Verification items for the finished model (mm, model axes). Face numbers are marked on the shaded views. A direction names the side the tool comes from. Coordinates: 2 decimals unless noted, no trailing zeros. Loops run counter-clockwise (first coordinate to the right, second up) from the corner with the lowest first, then second, coordinate; pieces in that order, holes last. Notation, with made-up numbers: (11, 12.5) -> (36, 12.5) arc R9 cw to (36, 22.5) -> close; hole circle Ø8 at (11, 6.25). An arc over 180 degrees is marked (long way). Answer as a JSON object with one key per item and string values. Group by question number.
Q1. Gauge pin test, flat ends, axial feed: pin 1 Ø5 at (y, z) = (-1, 4.5) entering from -X; pin 2 Ø1.5 at (y, z) = (-8, 7) entering from +X; pin 3 Ø4 at (y, z) = (-2.5, 2.5) entering from +X; pin 4 Ø3 at (y, z) = (-4, 12) entering from -X. Record the tip position at first contact, or that the pin passes through.
Q2. Set-up check for the marked faces 4 and 5: record each of +Z, -Z, +X, -X, +Y, -Y from which the full face is reachable in a straight line by a thin tool's end or side.
Q3. Release check for a two-part mould opening along Y. For the marked faces 1, 2 and 3 record: released by +Y, released by -Y, zero draft, split by the parting line, or undercut.
Q4. Cross-section at C-C on x = -165.5. Record the boundary of the cut face in (y, z).
Q5. Cross-section at A-A on y = 0.05. Record the boundary of the cut face in (x, z), and give its area (3 significant figures).
Q6. Scan lines: L1, parallel to Y at x = -94, z = 5; L2, parallel to X at y = 0.5, z = 4.25; L3, parallel to X at y = -8, z = 5.5. Record each from-to range of solid material in increasing order.
Q7. Cross-section at B-B on z = 8.75. Record the boundary of the cut face in (x, y).
```python
from build123d import *

# Parameters (mm, degrees)
SKETCH1_R          = 10
EXTRUDE1_DEPTH     = 15
CUT_EXTRUDE1_START = -15
CUT_EXTRUDE1_DEPTH = 15


# Read off the part's stored shape, not the designer's step: Cut-Extrude1
with BuildPart() as part:
    # Sketch1 → Extrude1 (new body)
    with BuildSketch(Plane.XY):
        with BuildLine():
            Line((-200, 15.05), (0, 15.05))
            ThreePointArc((0, 15.05), (15, 0.05), (0, -14.95))
            Line((0, -14.95), (-200, -14.95))
            ThreePointArc((-200, -14.95), (-215, 0.05), (-200, 15.05))
        make_face()
        with Locations((-200, 0.05)):
            Circle(SKETCH1_R, mode=Mode.SUBTRACT)
        Circle(SKETCH1_R, mode=Mode.SUBTRACT)
    extrude(amount=EXTRUDE1_DEPTH)

    # Cut-Extrude1 outline → Cut-Extrude1 (cut)
    with BuildSketch(Plane.XY.offset(15).offset(CUT_EXTRUDE1_START)):
        with BuildLine():
            ThreePointArc((-199.997500016, 10.049999688), (-190.000000313, 0.0475), (-200.002500016, -9.949999687))
            Line((-200.002500016, -9.949999687), (-0.002499984, -9.999999688))
            ThreePointArc((-0.002499984, -9.999999688), (-9.999999922, 0.001249992), (0, 10))
            Line((0, 10), (-199.997500016, 10.049999688))
        make_face()
    extrude(amount=CUT_EXTRUDE1_DEPTH, mode=Mode.SUBTRACT)


solid = part.part
```
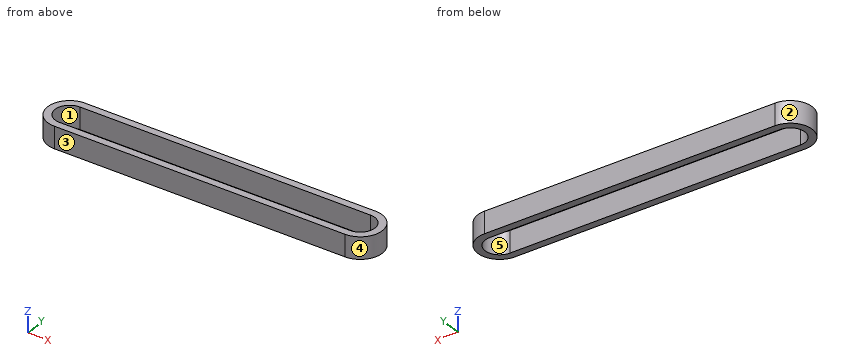
Computed values:
{
 "1": {"pin 1": "stops at x = -215", "pin 2": "stops at x = 13.1", "pin 3": "stops at x = 14.99", "pin 4": "stops at x = -214.78"},
 "2": {"face 4": "+Z, -Z, +X", "face 5": "+Z, -Z"},
 "3": {"face 1": "undercut", "face 2": "split by the parting line", "face 3": "released by -Y"},
 "4": {"outline": "(-14.95, 0) -> (-9.96, 0) -> (-9.96, 15) -> (-14.95, 15) -> close; (10.04, 0) -> (15.05, 0) -> (15.05, 15) -> (10.04, 15) -> close"},
 "5": {"outline": "(-215, 0) -> (-210, 0) -> (-210, 15) -> (-215, 15) -> close; (10, 0) -> (15, 0) -> (15, 15) -> (10, 15) -> close", "area": "150 mm²"},
 "6": {"L1": "y = -14.95 to -9.98, 10.02 to 15.05", "L2": "x = -214.99 to -209.99, 9.99 to 14.99", "L3": "x = -212.66 to -205.93, 6 to 12.66"},
 "7": {"outline": "(-200, -14.95) -> (0, -14.95) arc R15 ccw to (0, 15.05) -> (-200, 15.05) arc R15 ccw to start; hole (-200, -9.95) -> (0, -10) arc R10 ccw to (0, 10) -> (-200, 10.05) arc R10 ccw to start"}
}
